Here's how the part is built. I have some questions about the finished solid (model axes, mm). Face numbers are marked on the shaded views. Round coordinates to 2 decimals unless told otherwise and drop trailing zeros. Write each loop counter-clockwise with the first axis right and the second up, starting at its lowest first coordinate (ties: lowest second). Pieces come first, ordered by that corner, then holes. Notation, with made-up numbers: M 74,81.25 L 96,81.25 A24 ccw 96,120.25 Z; hole C -9.75,60 d8. An arc over 180 degrees is marked long. Use one line per item in the form item = value. Start each with the question number.
Q1. I want a section at D-D on z = 0.75. List the corners of the cut face in (x, y) for me, and give its area (3 significant figures).
Q2. I want a section at B-B on y = 7.5. List the corners of the cut face in (x, z) for me.
Q3. I want a section at A-A on z = 2.35. List the corners of the cut face in (x, y) for me, and give its area (3 significant figures).
Q4. We'd pull the mould along Y, two halves only. Please class the marked faces 1 and 2: +Y half, -Y half, draft (parallel to the pull), parting line (faces both ways), or undercut.
Q5. I want a section at C-C on x = 14. List the corners of the cut face in (y, z) for me.
Q6. I need wall thicknesses on line 1 along Y through (x, z) = (14, 0.65); line 2 along X through (y, z) = (-6, 2.15); line 3 along X through (y, z) = (6.5, 2.1). Which ranges of each line are inside material? Lowest first, please. Write a range as from..to.
Q7. I'm going to push flat-ended pins straight in: pin 1 Ø3.5 at (x, y) = (14, 7.5) entering from +Z; pin 2 Ø0.8 at (y, z) = (4, 2) entering from -X; pin 3 Ø0.8 at (x, z) = (1.5, 2.5) entering from +Y. Where does each tip first touch, or does it pass through?
```python
from build123d import *

# Parameters (mm, degrees)
SKETCH_1_W      = 34
SKETCH_1_H      = 21
SKETCH_1_R      = 1.5
EXTRUDE_1_DEPTH = 1.5
SKETCH_2_W      = 2.609332225
SKETCH_2_H      = 6.222253767
SKETCH_2_H_2    = 7.326202017
SKETCH_2_W_2    = 17.412274655
SKETCH_2_H_3    = 8.664478865
SKETCH_2_W_3    = 19.018017562
SKETCH_2_H_4    = 3.261665282
EXTRUDE_2_DEPTH = 1.5


with BuildPart() as part:
    # 草图1 → 凸台-拉伸1 (new body)
    with BuildSketch(Plane.XY):
        Rectangle(SKETCH_1_W, SKETCH_1_H)
        with Locations((14, 7.5)):
            Circle(SKETCH_1_R, mode=Mode.SUBTRACT)
        with Locations((14, -7.5)):
            Circle(SKETCH_1_R, mode=Mode.SUBTRACT)
    extrude(amount=EXTRUDE_1_DEPTH)

    # 草图2 → 凸台-拉伸2 (add)
    with BuildSketch(Plane.XY.offset(1.5)):
        with Locations((-14.208471454, 5.553351982)):
            Rectangle(SKETCH_2_W, SKETCH_2_H)
        with Locations((-14.208471454, -4.783617987)):
            Rectangle(SKETCH_2_W, SKETCH_2_H_2)
        with Locations((-0.032772348, 4.332239433)):
            Rectangle(SKETCH_2_W_2, SKETCH_2_H_3)
        with Locations((-0.835643802, -6.815886354)):
            Rectangle(SKETCH_2_W_3, SKETCH_2_H_4)
    extrude(amount=EXTRUDE_2_DEPTH)


solid = part.part
```
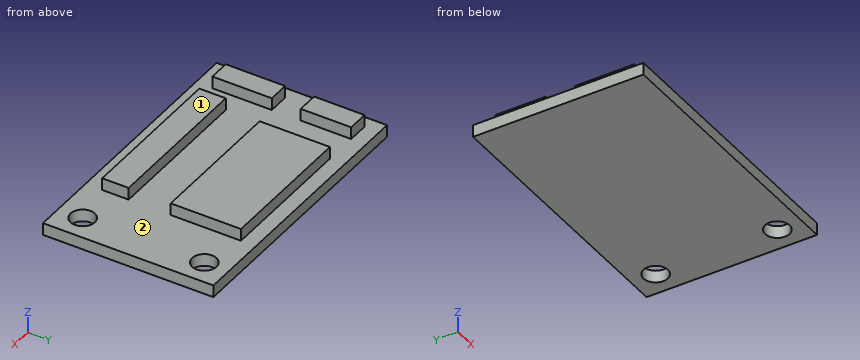
Reported:
q1.outline = M -17,-10.5 L 17,-10.5 L 17,10.5 L -17,10.5 Z; hole C 14,-7.5 d3; hole C 14,7.5 d3
q1.area = 700 mm^2
q2.outline = M -17,0 L 12.5,0 L 12.5,1.5 L 8.67,1.5 L 8.67,3 L -8.74,3 L -8.74,1.5 L -12.9,1.5 L -12.9,3 L -15.51,3 L -15.51,1.5 L -17,1.5 Z; M 15.5,0 L 17,0 L 17,1.5 L 15.5,1.5 Z
q3.outline = M -15.51,-8.45 L -12.9,-8.45 L -12.9,-1.12 L -15.51,-1.12 Z; M -15.51,2.44 L -12.9,2.44 L -12.9,8.66 L -15.51,8.66 Z; M -10.34,-8.45 L 8.67,-8.45 L 8.67,-5.19 L -10.34,-5.19 Z; M -8.74,0 L 8.67,0 L 8.67,8.66 L -8.74,8.66 Z
q3.area = 248 mm^2
q4.face_1 = draft
q4.face_2 = undercut
q5.outline = M -10.5,0 L -9,0 L -9,1.5 L -10.5,1.5 Z; M -6,0 L 6,0 L 6,1.5 L -6,1.5 Z; M 9,0 L 10.5,0 L 10.5,1.5 L 9,1.5 Z
q6.line_1 = -10.5..-9, -6..6, 9..10.5
q6.line_2 = -15.51..-12.9, -10.34..8.67
q6.line_3 = -15.51..-12.9, -8.74..8.67
q7.pin_1 = 1.5
q7.pin_2 = -15.51
q7.pin_3 = 8.66
